```python
from build123d import *

# Parameters (mm, degrees)
SKETCH1_W           = 38
SKETCH1_H           = 28
BOSS_EXTRUDE1_DEPTH = 1.5
SKETCH2_R           = 3.75
BOSS_EXTRUDE2_DEPTH = 8
SKETCH3_W           = 5.75
SKETCH3_H           = 6.25
BOSS_EXTRUDE3_DEPTH = 2.5
SKETCH4_W           = 16
SKETCH4_H           = 17
BOSS_EXTRUDE4_DEPTH = 2
SKETCH5_R           = 1
CUT_EXTRUDE1_DEPTH  = 2
SKETCH7_R           = 1
CUT_EXTRUDE3_DEPTH  = 2
SKETCH8_W           = 8
SKETCH8_H           = 20
BOSS_EXTRUDE5_DEPTH = 10.5
CHAMFER1_SIZE       = 5
CHAMFER1_SIZE2      = 1.819851171


with BuildPart() as part:
    # Sketch1 → Boss-Extrude1 (new body)
    with BuildSketch(Plane.XY):
        Rectangle(SKETCH1_W, SKETCH1_H)
    extrude(amount=BOSS_EXTRUDE1_DEPTH)

    # Sketch2 → Boss-Extrude2 (add)
    with BuildSketch(Plane.XY.offset(1.5)):
        with Locations((5, 8.75)):
            Circle(SKETCH2_R)
    extrude(amount=BOSS_EXTRUDE2_DEPTH)

    # Sketch3 → Boss-Extrude3 (add)
    with BuildSketch(Plane.XY.offset(1.5)):
        with Locations((-4.625, 9.375)):
            Rectangle(SKETCH3_W, SKETCH3_H)
    extrude(amount=BOSS_EXTRUDE3_DEPTH)

    # Sketch4 → Boss-Extrude4 (add)
    with BuildSketch(Plane.XY.offset(1.5)):
        with Locations((0.5, -5)):
            Rectangle(SKETCH4_W, SKETCH4_H)
    extrude(amount=BOSS_EXTRUDE4_DEPTH)

    # Sketch5 → Cut-Extrude1 (cut)
    with BuildSketch(Plane.XY.offset(1.5)):
        with Locations((14.5, -12.5)):
            Circle(SKETCH5_R)
    extrude(amount=-CUT_EXTRUDE1_DEPTH, mode=Mode.SUBTRACT)

    # Sketch7 → Cut-Extrude3 (cut)
    with BuildSketch(Plane.XY.offset(1.5)):
        with Locations((-17.5, 12.5)):
            Circle(SKETCH7_R)
    extrude(amount=-CUT_EXTRUDE3_DEPTH, mode=Mode.SUBTRACT)

    # Sketch8 → Boss-Extrude5 (add)
    with BuildSketch(Plane.XY.offset(1.5)):
        with Locations((-16.5, -4.1)):
            Rectangle(SKETCH8_W, SKETCH8_H)
    extrude(amount=BOSS_EXTRUDE5_DEPTH)

    # Chamfer1
    chamfer1_edges = [part.edges().sort_by_distance(p)[0] for p in [
        (-20.5, -4.1, 12),
    ]]
    chamfer1_side = [part.faces().sort_by_distance(p)[0] for p in [
        (-20.5, -4.1, 6.75),
    ]]
    chamfer(chamfer1_edges, length=CHAMFER1_SIZE, length2=CHAMFER1_SIZE2, reference=chamfer1_side[0])


solid = part.part
```
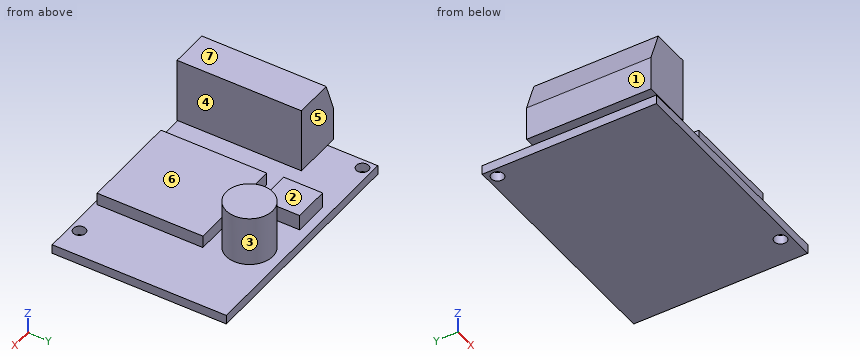
Part model, mm, in its own coordinate system. Face numbers are marked on the shaded views. A direction names the side the tool comes from. Coordinates: 2 decimals unless noted, no trailing zeros. Order: outer loops, then holes, each group sorted by start corner. A loop starts at its lowest first (then second) coordinate and runs counter-clockwise, first axis right, second up. Notation, with made-up numbers: (81, 53.5) -> (95, 53.5) arc R34 ccw to (95, 92.5) -> close; hole circle Ø11 at (78, -36). An arc over 180 degrees is marked (long way). Put each result on its own line as item: value. Start each with the question number.
(1) Band-saw the part on A-A (y = -12.5). Give the cut face in (x, z), then the cut area to 3 significant figures.
(2) Pin check, flat tips, straight feed: pin 1 Ø5 at (x, z) = (7, 6) entering from +Y; pin 2 Ø1 at (y, z) = (-3.5, 2.5) entering from +X; pin 3 Ø0.6 at (x, z) = (-2, 2.5) entering from -Y. Stop position of each tip, or through.
(3) Which spindle directions (+Z, -Z, +X, -X, +Y, -Y) get a long thin tool onto all of the face, cutting with end or side? Do the marked faces 4, 5, 6 and 7. Say none if no direction does.
(4) Band-saw the part on C-C (y = 8.75). Give the cut face in (x, z), then the cut area to 3 significant figures.
(5) Probe line 1 along Y through (x, z) = (-17.5, 0.6); line 2 along Y through (x, z) = (14.5, 1); line 3 along X through (y, z) = (-9.5, 3.25). List the from-to ranges inside material, lowest first. Write a range as [from, to].
(6) Band-saw the part on B-B (x = 14.5). Give the cut face in (y, z), then the cut area to 3 significant figures.
(7) Band-saw the part on D-D (x = -0.5). Give the cut face in (y, z).
(8) Mould opens along X. For the marked faces 1, 2 and 3 say: pulls with the +X half, pulls with the -X half, needs draft (parallel to the pull), parting line crosses it, or undercut.
Determined:
1. outline: (-20.5, 1.5) -> (-19, 1.5) -> (-19, 0) -> (13.5, 0) -> (13.5, 1.5) -> (8.5, 1.5) -> (8.5, 3.5) -> (-7.5, 3.5) -> (-7.5, 1.5) -> (-12.5, 1.5) -> (-12.5, 12) -> (-18.68, 12) -> (-20.5, 7) -> close; (15.5, 0) -> (19, 0) -> (19, 1.5) -> (15.5, 1.5) -> close
1. area: 165 mm²
2. pin 1: stops at y = 12.5
2. pin 2: stops at x = 8.5
2. pin 3: stops at y = -13.5
3. face 4: +Z, +Y, -Y
3. face 5: +Z, -X, +Y
3. face 6: +Z, +X, -Y
3. face 7: +Z, +X, -X, +Y, -Y
4. outline: (-19, 0) -> (19, 0) -> (19, 1.5) -> (8.75, 1.5) -> (8.75, 9.5) -> (1.25, 9.5) -> (1.25, 1.5) -> (-1.75, 1.5) -> (-1.75, 4) -> (-7.5, 4) -> (-7.5, 1.5) -> (-19, 1.5) -> close
4. area: 131 mm²
5. line 1: y = [-14, 11.5], [13.5, 14]
5. line 2: y = [-14, -13.5], [-11.5, 14]
5. line 3: x = [-20.5, -12.5], [-7.5, 8.5]
6. outline: (-14, 0) -> (-13.5, 0) -> (-13.5, 1.5) -> (-14, 1.5) -> close; (-11.5, 0) -> (14, 0) -> (14, 1.5) -> (-11.5, 1.5) -> close
6. area: 39.0 mm²
7. outline: (-14, 0) -> (14, 0) -> (14, 1.5) -> (3.5, 1.5) -> (3.5, 3.5) -> (-13.5, 3.5) -> (-13.5, 1.5) -> (-14, 1.5) -> close
8. face 1: pulls with the -X half
8. face 2: needs draft
8. face 3: undercut
